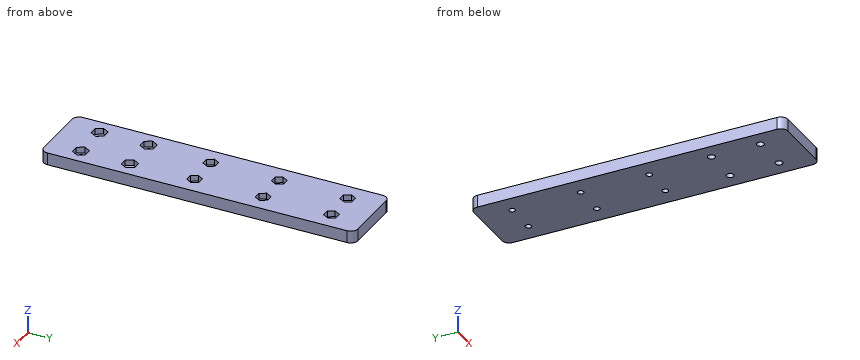
from build123d import *

# Parameters (mm, degrees)
F0_W     = 28.5
F0_H     = 128.5
F0_R     = 1.5
F0_R_2   = 1.25
F1_DEPTH = 5
F2_R     = 1.25
F2_R_2   = 1.5
F3_DEPTH = 2.4
F4_R     = 3


with BuildPart() as f1:
    # F0 (on Top) → F1 (new body)
    with BuildSketch(Plane.XY):
        with Locations((14.25, 64.25)):
            Rectangle(F0_W, F0_H)
        with Locations((6.75, 13.25)):
            Circle(F0_R, mode=Mode.SUBTRACT)
        with Locations((6.75, 33.25)):
            Circle(F0_R, mode=Mode.SUBTRACT)
        with Locations((7.75, 59.25)):
            Circle(F0_R_2, mode=Mode.SUBTRACT)
        with Locations((21.75, 13.25)):
            Circle(F0_R, mode=Mode.SUBTRACT)
        with Locations((20.75, 59.25)):
            Circle(F0_R_2, mode=Mode.SUBTRACT)
        with Locations((21.75, 33.25)):
            Circle(F0_R, mode=Mode.SUBTRACT)
        with Locations((7.75, 87.25)):
            Circle(F0_R_2, mode=Mode.SUBTRACT)
        with Locations((7.75, 115.25)):
            Circle(F0_R_2, mode=Mode.SUBTRACT)
        with Locations((20.75, 87.25)):
            Circle(F0_R_2, mode=Mode.SUBTRACT)
        with Locations((20.75, 115.25)):
            Circle(F0_R_2, mode=Mode.SUBTRACT)
    extrude(amount=F1_DEPTH)

    # F2 (on face) → F3 (cut)
    with BuildSketch(Plane.XY.offset(5)):
        Polygon((6.306624, 84.75), (9.193376, 84.75), (10.636751, 87.25), (9.193376, 89.75), (6.306624, 89.75), (4.863249, 87.25), align=None)
        with Locations((7.75, 87.25)):
            Circle(F2_R, mode=Mode.SUBTRACT)
        Polygon((19.306624, 84.75), (22.193376, 84.75), (23.636751, 87.25), (22.193376, 89.75), (19.306624, 89.75), (17.863249, 87.25), align=None)
        with Locations((20.75, 87.25)):
            Circle(F2_R, mode=Mode.SUBTRACT)
        Polygon((6.306624, 112.75), (9.193376, 112.75), (10.636751, 115.25), (9.193376, 117.75), (6.306624, 117.75), (4.863249, 115.25), align=None)
        with Locations((7.75, 115.25)):
            Circle(F2_R, mode=Mode.SUBTRACT)
        Polygon((19.306624, 112.75), (22.193376, 112.75), (23.636751, 115.25), (22.193376, 117.75), (19.306624, 117.75), (17.863249, 115.25), align=None)
        with Locations((20.75, 115.25)):
            Circle(F2_R, mode=Mode.SUBTRACT)
        Polygon((19.306624, 56.75), (22.193376, 56.75), (23.636751, 59.25), (22.193376, 61.75), (19.306624, 61.75), (17.863249, 59.25), align=None)
        with Locations((20.75, 59.25)):
            Circle(F2_R, mode=Mode.SUBTRACT)
        Polygon((6.306624, 56.75), (9.193376, 56.75), (10.636751, 59.25), (9.193376, 61.75), (6.306624, 61.75), (4.863249, 59.25), align=None)
        with Locations((7.75, 59.25)):
            Circle(F2_R, mode=Mode.SUBTRACT)
        Polygon((5.162287, 30.5), (8.337713, 30.5), (9.925426, 33.25), (8.337713, 36), (5.162287, 36), (3.574574, 33.25), align=None)
        with Locations((6.75, 33.25)):
            Circle(F2_R_2, mode=Mode.SUBTRACT)
        Polygon((20.162287, 10.5), (23.337713, 10.5), (24.925426, 13.25), (23.337713, 16), (20.162287, 16), (18.574574, 13.25), align=None)
        with Locations((21.75, 13.25)):
            Circle(F2_R_2, mode=Mode.SUBTRACT)
        Polygon((5.162287, 10.5), (8.337713, 10.5), (9.925426, 13.25), (8.337713, 16), (5.162287, 16), (3.574574, 13.25), align=None)
        with Locations((6.75, 13.25)):
            Circle(F2_R_2, mode=Mode.SUBTRACT)
        Polygon((20.162287, 30.5), (23.337713, 30.5), (24.925426, 33.25), (23.337713, 36), (20.162287, 36), (18.574574, 33.25), align=None)
        with Locations((21.75, 33.25)):
            Circle(F2_R_2, mode=Mode.SUBTRACT)
    extrude(amount=-F3_DEPTH, mode=Mode.SUBTRACT)

    # F4
    f4_edges = [f1.edges().sort_by_distance(p)[0] for p in [
        (0, 0, 2.5),
        (28.5, 0, 2.5),
        (0, 128.5, 2.5),
        (28.5, 128.5, 2.5),
    ]]
    fillet(f4_edges, radius=F4_R)


solid = f1.part
Read the model definition and answer for the solid it produces. Units are mm, in the model's axes. Coordinates: 2 decimals unless noted, no trailing zeros. Use a Markdown table: item, result.
Q1. The part is cut by section A-A, the plane z = 0.8. Give the number of separate pieces and of enclosed holes in the cut face, then the cut area to 3 significant figures.
Answer block:
| item | result |
|---|---|
| separate pieces | 1 |
| enclosed holes | 10 |
| area | 3,600 mm2 |
Q2. Each of these flat-tipped pins is pushed along its axis until it touches: pin 1 Ø1.5 at (x, y) = (8, 115) entering from +Z; pin 2 Ø2.5 at (x, y) = (19.5, 87.5) entering from +Z. Where does it stop, or does it pass through?
Answer block:
| item | result |
|---|---|
| pin 1 | passes through |
| pin 2 | stops at z = 2.6 |
Q3. Straight lines are drawn through the part: L1, parallel to Y at x = 6.5, z = 3.4; L2, parallel to X at y = 115.25, z = 1.25; L3, parallel to Y at x = 18, z = 4.4. For each, find the intervals that lie inside material, in ascending order. Write a range as [from, to].
Answer block:
| item | result |
|---|---|
| L1 | y = [0, 10.5], [16, 30.5], [36, 56.75], [61.75, 84.75], [89.75, 112.75], [117.75, 128.5] |
| L2 | x = [0, 6.5], [9, 19.5], [22, 28.5] |
| L3 | y = [0, 59.01], [59.49, 87.01], [87.49, 115.01], [115.49, 128.5] |
